Input: part model. Units: mm. Frame: model coordinates. Face numbers are marked on the shaded views. A direction names the side the tool comes from. Round coordinates to 2 decimals unless told otherwise and drop trailing zeros. Loops run counter-clockwise (first coordinate to the right, second up) from the corner with the lowest first, then second, coordinate; pieces in that order, holes last. Notation, with made-up numbers: M -2.75,-5 L 50.25,-5 A26 ccw 50.25,24 Z; hole C 22,-5.75 d2. An arc over 180 degrees is marked long. Return JSON: item names as keys, results as strings. Group by question number.
1) Section C-C (y = 42). Count the separate pieces of the cut face and the enclosed holes in it, plus the area to 3 significant figures.
2) Section A-A (x = -76.2). Output: boundary loops of the cut face in (y, z) (3 decimals), plus the area to 3 significant figures.
3) Access query for the marked faces 5, 6 and 7. Directions: +Z, -Z, +X, -X, +Y, -Y. A direction counts if a zero-diameter tool reaches every point of the face in a straight line with its end or side. Return the directions, or none.
4) Section B-B (z = -5). Output: boundary loops of the cut face in (x, y) (3 decimals).
5) Contact query for flat-ended pins moving along their axis: P1, Ø22, axis at x = 76.2, y = 38.1, coming from the +Z side; P2, Ø3, axis at x = -49, y = 33.5, coming from the +Z side; P3, Ø1.5, axis at x = -2.5, y = 23.5, coming from the -Z side. Output: stop coordinate, or through.
6) Material intervals for line 1 (X direction, y = 38, z = 8); line 2 (Y direction, x = 76.2, z = 4.5) (3 decimals); line 3 (X direction, y = 38.1, z = 5.75) (3 decimals), sorted ascending. Write a range as from..to.
7) Mould query, pull axis Y, two halves, no side actions, for the marked faces 1, 2, 3 and 4. Classes: +Y half, -Y half, draft (parallel to the pull), parting line (faces both ways), or undercut.
Autodesk Inventor part; units mm, degrees
ref_plane "YZ Plane" through (0, 0, 0) normal (1, 0, 0) x (0, 1, 0)
ref_plane "XZ Plane" through (0, 0, 0) normal (0, 1, 0) x (-1, 0, 0)
ref_plane "XY Plane" through (0, 0, 0) normal (0, 0, 1) x (1, 0, 0)
sketch "Sketch1" plane through (0, 0, 0) normal (0, 1, 0) x (-1, 0, 0)
  line L0 (98.425, 0) -> (98.425, -19.05)
  line L1 (98.425, -19.05) -> (111.125, -19.05)
  line L2 (111.125, -19.05) -> (111.125, 12.7)
  line L3 (111.125, 12.7) -> (46.0322, 12.7)
  arc A0 (35.052, 0) -> (0, 35.052) centre (0, 0) ccw
  line L4 (0, 0) -> (35.052, 0) construction
  line L5 (0, 0) -> (35.052, 0) construction
  line L6 (0, 0) -> (0, 47.752) construction
  arc A1 (46.0322, 12.7) -> (0, 47.752) centre (0, 0) ccw
  line L7 (35.052, 0) -> (98.425, 0)
  line L8 (-98.425, 0) -> (-98.425, -19.05)
  line L9 (-98.425, -19.05) -> (-111.125, -19.05)
  line L10 (-111.125, -19.05) -> (-111.125, 12.7)
  line L11 (-111.125, 12.7) -> (-46.0322, 12.7)
  arc A2 (0, 35.052) -> (-35.052, 0) centre (0, 0) ccw
  arc A3 (0, 47.752) -> (-46.0322, 12.7) centre (0, 0) ccw
  line L12 (-35.052, 0) -> (-98.425, 0)
  arc A4 (35.052, 0) -> (-35.052, 0) centre (0, 0) ccw
  arc A5 (46.0322, 12.7) -> (-46.0322, 12.7) centre (0, 0) ccw
  line L13 (35.052, 0) -> (98.425, 0)
  line L14 (98.425, 0) -> (98.425, -19.05)
  line L15 (111.125, -19.05) -> (111.125, 12.7)
  line L16 (46.0322, 12.7) -> (111.125, 12.7)
  line L17 (-46.0322, 12.7) -> (-111.125, 12.7)
  line L18 (-111.125, -19.05) -> (-111.125, 12.7)
  line L19 (-98.425, -19.05) -> (-111.125, -19.05)
  line L20 (-98.425, 0) -> (-35.052, 0)
  line L21 (-98.425, 0) -> (-35.052, 0)
  dimension "d7" = 12.7
  dimension "d9" = 35.052
  dimension "d10" = 0
  dimension "d11" = 90
  dimension "d12" = 12.7
  dimension "d13" = 31.75
  dimension "d14" = 12.7
  dimension "d30" = 98.425
extrude "Extrusion1" add sketch "Sketch1" along normal blind 76.2
fillet "Fillet1" radius 9.652 8 edges at (111.125, 38.1, 12.7) (46.0322, 38.1, 12.7) (104.775, 76.2, -19.05) (104.775, 0, -19.05) (-46.0322, 38.1, 12.7) (-111.125, 38.1, 12.7) (-104.775, 0, -19.05) (-104.775, 76.2, -19.05)
sketch "Sketch2" plane through (52.8735, 0, 12.7) normal (0, 0, 1) x (1, 0, 0)
  line L0 (-52.8735, 0) -> (-52.8735, 38.1) construction
  line L1 (-52.8735, 38.1) -> (-129.0735, 38.1) construction
  line L2 (-52.8735, 38.1) -> (23.3265, 38.1) construction
  dimension "d20" = 38.1
  dimension "d21" = 76.2
  dimension "d22" = 76.2
hole "Hole1" at (-76.2, 38.1, 12.7) at (76.2, 38.1, 12.7) direction (0, 0, -1) diameter 19.05 end through all
properties part number "SólidoA"
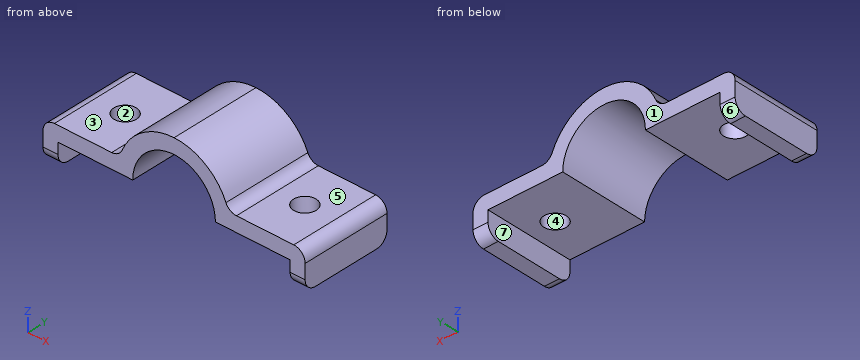
Returned:
{
 "1": {"separate pieces": "3", "enclosed holes": "0", "area": "3,290 mm^2"},
 "2": {"outline": "M 0,0 L 28.575,0 L 28.575,12.7 L 0,12.7 Z; M 47.625,0 L 76.2,0 L 76.2,12.7 L 47.625,12.7 Z", "area": "726 mm^2"},
 "3": {"face 5": "+Z, +X, +Y, -Y", "face 6": "-Z, +X, -X, +Y", "face 7": "-Z, +Y, -Y"},
 "4": {"outline": "M -111.125,0 L -98.425,0 L -98.425,76.2 L -111.125,76.2 Z; M 98.425,0 L 111.125,0 L 111.125,76.2 L 98.425,76.2 Z"},
 "5": {"P1": "stops at z = 12.7", "P2": "stops at z = 14.33", "P3": "stops at z = 34.9"},
 "6": {"line 1": "x = -109.76..-85.72, -66.68..-34.13, 34.13..66.68, 85.72..109.76", "line 2": "y = 0..28.575, 47.625..76.2", "line 3": "x = -110.739..-85.725, -66.675..-34.577, 34.577..66.675, 85.725..110.739"},
 "7": {"face 1": "+Y half", "face 2": "undercut", "face 3": "draft", "face 4": "undercut"}
}
